Autodesk Inventor part; units mm, degrees
ref_plane "YZ Plane" through (0, 0, 0) normal (1, 0, 0) x (0, 1, 0)
ref_plane "XZ Plane" through (0, 0, 0) normal (0, 1, 0) x (-1, 0, 0)
ref_plane "XY Plane" through (0, 0, 0) normal (0, 0, 1) x (1, 0, 0)
sketch "Эскиз1" plane through (0, 0, 0) normal (0, 0, 1) x (1, 0, 0)
  arc A0 (6.1718, 12.1916) -> (6.0205, -0.0083) centre (6, 6.0928) ccw
  line L0 (6.1718, 12.1916) -> (6.0205, -0.0083) construction
  line L1 (6.1718, 12.1916) -> (18.3727, 12.1916) construction
  arc A1 (42.148, 8.0153) -> (37.9718, 12.1916) centre (37.9718, 8.0153) ccw
  arc A2 (37.8204, -0.0083) -> (42.148, 4.3193) centre (37.8204, 4.3193) ccw
  arc A3 (6.1001, 13.1916) -> (6.1001, -1.0083) centre (6.1001, 6.0916) ccw
  arc A4 (43.148, 7.5237) -> (37.78, 13.1916) centre (37.4718, 7.5237) ccw
  arc A5 (37.7733, -1.0083) -> (43.148, 4.6599) centre (37.4718, 4.6599) ccw
  line L2 (6.1718, 12.1916) -> (37.9718, 12.1916)
  line L3 (37.78, 13.1916) -> (6.1001, 13.1916)
  line L4 (6.0205, -0.0083) -> (37.8204, -0.0083)
  line L5 (37.7733, -1.0083) -> (6.1001, -1.0083)
  line L6 (42.148, 8.0153) -> (42.148, 4.3193)
  line L7 (43.148, 7.5237) -> (43.148, 4.6599)
  point P0 (0, 0)
  point P1 (0, 0)
  dimension "d7" = 1.5
  dimension "d0" = 90.71
  dimension "d1" = 4.1763
  dimension "d2" = 5.6763
  dimension "d3" = 5.6763
  dimension "d4" = 1
  dimension "d5" = 1
  dimension "d8" = 12.1999
  dimension "d9" = 31.8
  dimension "d10" = 31.7998
  dimension "d13" = 1
extrude "main_walls" add sketch "Эскиз1" along normal blind 6
sketch "Эскиз2" plane through (0, 0, 0) normal (0, 0, -1) x (-1, 0, 0)
  line L0 (-37.7733, -1.0083) -> (-6.1001, -1.0083)
  arc A0 (-6.1001, -1.0083) -> (-6.1001, 13.1916) centre (-6.1001, 6.0916) ccw
  line L1 (-6.1001, 13.1916) -> (-37.78, 13.1916)
  arc A1 (-37.78, 13.1916) -> (-43.148, 7.5237) centre (-37.4718, 7.5237) ccw
  line L2 (-43.148, 7.5237) -> (-43.148, 4.6599)
  arc A2 (-43.148, 4.6599) -> (-37.7733, -1.0083) centre (-37.4718, 4.6599) ccw
  point P0 (0, 0)
extrude "floor" add sketch "Эскиз2" along normal blind 1
sketch "Эскиз3" plane through (0, 0, 0) normal (0, 0, 1) x (1, 0, 0)
  line L0 (42.148, 4.3193) -> (42.148, 8.0153)
  arc A0 (42.148, 8.0153) -> (37.9718, 12.1916) centre (37.9718, 8.0153) ccw
  line L1 (37.9718, 12.1916) -> (6.1718, 12.1916)
  arc A1 (6.1718, 12.1916) -> (6.0205, -0.0083) centre (6, 6.0928) ccw
  line L2 (6.0205, -0.0083) -> (37.8204, -0.0083)
  arc A2 (37.8204, -0.0083) -> (42.148, 4.3193) centre (37.8204, 4.3193) ccw
  line L3 (-0.1012, 8.3416) -> (1.8988, 8.3416)
  line L4 (1.8988, 8.3416) -> (1.8988, 3.8416)
  line L5 (1.8988, 3.8416) -> (-0.1012, 3.8416)
  line L6 (-0.1012, 3.8416) -> (-0.1012, 8.3416)
  arc A3 (6.1718, 12.1916) -> (6.0205, -0.0083) centre (6, 6.0928) ccw
  arc A4 (42.148, 8.0153) -> (37.9718, 12.1916) centre (37.9718, 8.0153) ccw
  line L7 (6.1718, 12.1916) -> (37.9718, 12.1916)
  arc A5 (37.8204, -0.0083) -> (42.148, 4.3193) centre (37.8204, 4.3193) ccw
  line L8 (6.0205, -0.0083) -> (37.8204, -0.0083)
  line L9 (36.948, 12.1916) -> (39.448, 12.1916)
  line L10 (39.448, 12.1916) -> (39.448, -0.0083)
  line L11 (39.448, -0.0083) -> (36.948, -0.0083)
  line L12 (36.948, -0.0083) -> (36.948, 12.1916)
  point P0 (0, 0)
  dimension "d16" = 2
  dimension "d17" = 4.5
  dimension "d18" = 12.1999
  dimension "d19" = 3.85
  dimension "d22" = 2.7
  dimension "d23" = 2.5
extrude "supports" add sketch "Эскиз3" along normal blind 4 contours L10 L11 A2 | A2 L2 L12 L1 A0 L10 | A0 L9 L10 | L5 L6 A1 | A1 L3 L4 L5 | A1 L6 L3
fillet "bottom_rounding" radius 1 13 edges at (21.5599, 12.1916, 0) (21.4843, -0.0083, 0) (2.5814, 1.0393, 0) (2.6433, 11.1876, 0) (42.148, 6.1673, 0) (41.4101, 1.9022, 0) (41.4073, 10.3898, 0) (-0.9999, 6.0916, -1) (21.94, 13.1916, -1) (21.9367, -1.0083, -1) (43.148, 6.0918, -1) (41.593, 11.4269, -1) (41.5907, 0.7543, -1)
sketch "Эскиз5" plane through (0, 0, 0) normal (0, 0, 1) x (1, 0, 0)
  arc A0 (1.4224, 3.8416) -> (6.0188, 0.9917) centre (6, 6.0928) ccw
  line L0 (36.948, 0.9917) -> (6.0188, 0.9917)
  line L1 (36.948, 0.9917) -> (36.948, 11.1916)
  line L2 (6.1571, 11.1916) -> (36.948, 11.1916)
  arc A1 (6.1571, 11.1916) -> (1.4212, 8.3416) centre (6, 6.0928) ccw
  line L3 (1.4212, 8.3416) -> (1.8988, 8.3416)
  line L4 (1.8988, 8.3416) -> (1.8988, 3.8416)
  line L5 (1.8988, 3.8416) -> (1.4224, 3.8416)
  line L6 (9.8988, 0.9917) -> (9.8988, 11.1916)
  point P0 (0, 0)
  dimension "d27" = 8
sketch "Эскиз6" plane through (0, 0, -1) normal (0, 0, -1) x (-1, 0, 0)
  line L0 (-1.8988, 8.3416) -> (-1.8988, 3.8416)
  line L1 (-1.4212, 8.3416) -> (-1.8988, 8.3416)
  arc A0 (-1.4212, 8.3416) -> (-6.1571, 11.1916) centre (-6, 6.0928) ccw
  line L2 (-1.8988, 3.8416) -> (-1.4224, 3.8416)
  arc A1 (-6.0188, 0.9917) -> (-1.4224, 3.8416) centre (-6, 6.0928) ccw
  line L3 (-6.1001, -0.0083) -> (-37.7455, -0.0083)
  arc A2 (-6.1001, -0.0083) -> (-6.1001, 12.1916) centre (-6.1001, 6.0916) ccw
  line L4 (-37.7515, 12.1916) -> (-6.1001, 12.1916)
  arc A3 (-37.7515, 12.1916) -> (-42.148, 7.5237) centre (-37.4718, 7.5237) ccw
  line L5 (-42.148, 4.6599) -> (-42.148, 7.5237)
  arc A4 (-42.148, 4.6599) -> (-37.7455, -0.0083) centre (-37.4718, 4.6599) ccw
  line L6 (-6.1571, 11.1916) -> (-36.948, 11.1916)
  line L7 (-36.948, 0.9917) -> (-6.0188, 0.9917)
  line L8 (-11.8741, 11.1916) -> (-11.8741, 0.9917)
  line L9 (-3.8741, 10.7299) -> (-3.8741, 1.4557)
  line L10 (-6.1001, 13.1916) -> (-37.78, 13.1916)
  line L11 (-3.8741, 10.7299) -> (-11.8741, 10.7299)
  line L12 (-11.8741, 10.7299) -> (-11.8741, 13.1916)
  line L13 (-11.8741, 13.1916) -> (-3.8741, 13.1916)
  line L14 (-3.8741, 13.1916) -> (-3.8741, 10.7299)
  point P0 (0, 0)
  dimension "d31" = 8
extrude "Выдавливание5" cut sketch "Эскиз6" against normal blind 5 contours L11 L8 L6 A0 | L9 A1 L7 L8 L11 | A0 L6 L12 L4 A2 L14 | A2 L4 L12 L10 L13 L14
equation "\"d2\" = d1 + d7"
equation "\"d3\" = d1 + d7"
equation "\"d5\" = d4"
equation "\"d13\" = d4"
equation "\"d19\" = -0.5 * d17 + 0.5 * d18"
properties part number "bottom"
Source: CAD feature listing. Evaluate the final solid. Frame: model axes, mm. A direction names the side the tool comes from. Coordinates: 2 decimals unless noted, no trailing zeros. Loops run counter-clockwise (first coordinate to the right, second up) from the corner with the lowest first, then second, coordinate; pieces in that order, holes last. Notation, with made-up numbers: (39.25, -21.5) -> (73.25, -21.5) arc R22 ccw to (73.25, 17.5) -> close; hole circle Ø8 at (-15.5, 52.25). An arc over 180 degrees is marked (long way). Answer in a Markdown table with one row per item. Add a question column.
Q1. Section B-B on z = 2.25. Return the cut outline in (x, y).
Q2. Ray query, line 1 along Y through (x, z) = (35, 4.75); line 2 along X through (y, z) = (8.75, 3.5); line 3 along X through (y, z) = (9, 1). Return the intervals inside material, ascending.
Q3. Pull-direction query (X, two-part tool) for faces 1 (the face through (21, 6, -1)), 2 (the face through (41.55, 11.47, 2.96)), 3 (the face through (1, 3.842, 2)); classes: pulls with the +X half, pulls with the -X half, needs draft (parallel to the pull), parting line crosses it, or undercut.
Q4. Reachability of faces 4 (the face through (25.008, 12.891, -0.715)), 5 (the face through (11.874, 8.9, -0.2)), 6 (the face through (9, 0.992, -0.5)), 7 (the face through (38, 6, 4)) from +Z, -Z, +X, -X, +Y, -Y: full face, straight path, thin tool, end or side. Return the list, or none.
Q5. Contact query for flat-ended pins moving along their axis: pin 1 Ø1.2 at (x, y) = (38.5, 7) entering from +Z; pin 2 Ø0.5 at (x, y) = (40.5, 7.5) entering from +Z; pin 3 Ø0.8 at (x, z) = (1, 2) entering from -Y; pin 4 Ø4 at (y, z) = (5.5, 2.5) entering from -X. Output: stop coordinate, or through.
Q6. Section C-C on x = 33. Return the cut outline in (y, z).
Q7. Section A-A on x = 7. Return the cut outline in (y, z).
Computed values:
| question | item | result |
|---|---|---|
| 1 | outline | (0.33, 3.84) -> (1.9, 3.84) -> (1.9, 8.34) -> (0.33, 8.34) arc R6.1 cw to (3.87, 11.81) -> (3.87, 12.83) arc R7.1 ccw to (6.1, -1.01) -> (37.77, -1.01) arc R5.68 ccw to (43.15, 4.66) -> (43.15, 7.52) arc R5.68 ccw to (37.78, 13.19) -> (11.87, 13.19) -> (11.87, 12.19) -> (36.95, 12.19) -> (36.95, -0.01) -> (6.02, -0.01) arc R6.1 cw to start; hole (39.45, 0.31) arc R4.33 ccw to (42.15, 4.32) -> (42.15, 8.02) arc R4.18 ccw to (39.45, 11.92) -> close |
| 2 | line 1 | y = -1.01 to -0.01, 12.19 to 13.19 |
| 2 | line 2 | x = -0.48 to 0.51, 36.95 to 39.45, 42.08 to 43.01 |
| 2 | line 3 | x = -0.38 to 0.64, 36.95 to 39.45, 42.03 to 42.95 |
| 3 | face 1 | needs draft |
| 3 | face 2 | pulls with the +X half |
| 3 | face 3 | undercut |
| 4 | face 4 | -Z, +X, -X, +Y |
| 4 | face 5 | -Z, +Y |
| 4 | face 6 | +Z, -Z, +Y |
| 4 | face 7 | +Z |
| 5 | pin 1 | stops at z = 4 |
| 5 | pin 2 | stops at z = 0 |
| 5 | pin 3 | stops at y = 0.77 |
| 5 | pin 4 | stops at x = -1 |
| 6 | outline | (-1.01, 0) arc R1 ccw to (-0.01, -1) -> (12.19, -1) arc R1 ccw to (13.19, 0) -> (13.19, 6) -> (12.19, 6) -> (12.19, 1) arc R1 cw to (11.19, 0) -> (0.99, 0) arc R1 cw to (-0.01, 1) -> (-0.01, 6) -> (-1.01, 6) -> close |
| 7 | outline | (-1.01, 0) arc R1 ccw to (-0.01, -1) -> (0.99, -1) -> (0.99, 0) arc R1 cw to (-0.01, 1) -> (-0.01, 6) -> (-1.01, 6) -> close; (12.19, 4) -> (13.19, 4) -> (13.19, 6) -> (12.19, 6) -> close |
